Work out the finished part from the listing and answer in its coordinate system (mm). A direction names the side the tool comes from. Give positions to 0.01 mm unless a question says otherwise; leave off trailing zeros. Write each loop counter-clockwise with the first axis right and the second up, starting at its lowest first coordinate (ties: lowest second). Pieces come first, ordered by that corner, then holes.
1) Determine the mould class of faces 1 (the face through (-119.425, 112.175, 151.445)), 2 (the face through (-290.34, 195.39, 144.21)), 3 (the face through (6.177, -11.876, 49.783)), 4 (the face through (-272.86, 177.91, 127.75)) for opening direction Z: pulls with the +Z half, pulls with the -Z half, needs draft (parallel to the pull), parting line crosses it, or undercut.
2) Find section A-A (z = 58). Determine the outline of the cut face in (x, y).
3) Straight lines are drawn through the part: probe 1 along Y at (x, z) = (0, 34); probe 2 along X at (y, z) = (184.5, 133.5). For each, find the intervals that lie inside material, in ascending order.
4) A tool of negligible diameter and unlimited length cuts with its end or side. For faces 5 (the face through (-1, -14, 0)), 6 (the face through (16, 5, 50)), from which of +Z, -Z, +X, -X, +Y, -Y can it reach the whole face along a straight path? Write none if from no direction.
5) Given pin 1 Ø1 at (x, z) = (-27.5, 132) entering from -Y; pin 2 Ø6 at (x, y) = (-197, 204.5) entering from -Z (3 decimals), each flat-ended and moving along its own axis, determine where each tip first touches the part or whether it passes through.
```python
from build123d import *

# Parameters (mm, degrees)
PIPESKETCH_R    = 16.764
PIPESKETCH_R_2  = 13.3858
EXTRUSION_DEPTH = 95
SKETCH_3_R      = 16.764
SKETCH_3_R_2    = 13.3858
EXTRUDE_2_DEPTH = 5.980008255
SKETCH_4_R      = 16.764
SKETCH_4_R_2    = 13.3858
REVOLVE_2_ANGLE = 90
SKETCH_5_R      = 16.764
SKETCH_5_R_2    = 13.3858
EXTRUDE_3_DEPTH = 254.900237781
SKETCH_6_R      = 16.764
SKETCH_6_R_2    = 13.3858
REVOLVE_3_ANGLE = 90
SKETCH_7_R      = 16.764
SKETCH_7_R_2    = 13.3858
EXTRUDE_4_DEPTH = 58.9


with BuildPart() as part:
    # PipeSketch → Extrusion (new body)
    with BuildSketch(Plane.XY):
        Circle(PIPESKETCH_R)
        Circle(PIPESKETCH_R_2, mode=Mode.SUBTRACT)
    extrude(amount=EXTRUSION_DEPTH)

    # 草图3 → 凸台-拉伸2 (add)
    with BuildSketch(Plane.XY.offset(95)):
        Circle(SKETCH_3_R)
        Circle(SKETCH_3_R_2, mode=Mode.SUBTRACT)
    extrude(amount=EXTRUDE_2_DEPTH)

    # 草图4 → 旋转2 (revolve)
    with BuildSketch(Plane.XY.offset(100.980008255)):
        with Locations(Location((0, 0, 0), (0, 0, 315))):
            Circle(SKETCH_4_R)
        with Locations(Location((0, 0, 0), (0, 0, 315))):
            Circle(SKETCH_4_R_2, mode=Mode.SUBTRACT)
    revolve(axis=Axis((-26.940768363, 26.940768363, 100.980008255), (-0.7071067811865476, -0.7071067811865476, 0)), revolution_arc=REVOLVE_2_ANGLE)

    # 草图5 → 凸台-拉伸3 (add)
    with BuildSketch(Plane(origin=(-26.940768363, 26.940768363, 0), x_dir=(0.7071067811865475, 0.7071067811865477, 0), z_dir=(-0.7071067811865477, 0.7071067811865475, 0))):
        with Locations(Location((0, -139.080008255, 0), (0, 0, 270))):
            Circle(SKETCH_5_R)
        with Locations(Location((0, -139.080008255, 0), (0, 0, 270))):
            Circle(SKETCH_5_R_2, mode=Mode.SUBTRACT)
    extrude(amount=EXTRUDE_3_DEPTH)

    # 草图6 → 旋转3 (revolve)
    with BuildSketch(Plane(origin=(-207.182455024, 207.182455024, 0), x_dir=(0, 0, 1), z_dir=(-0.7071067811865476, 0.7071067811865476, 0))):
        with Locations(Location((139.080008255, 0, 0), (0, 0, 90))):
            Circle(SKETCH_6_R)
        with Locations(Location((139.080008255, 0, 0), (0, 0, 90))):
            Circle(SKETCH_6_R_2, mode=Mode.SUBTRACT)
    revolve(axis=Axis((-234.123223388, 180.241686661, 139.080008255), (0, 0, 1)), revolution_arc=REVOLVE_3_ANGLE)

    # 草图7 → 凸台-拉伸4 (add)
    with BuildSketch(Plane(origin=(-26.940768363, -26.940768363, 0), x_dir=(-0.7071067811865479, 0.7071067811865472, 0), z_dir=(-0.7071067811865472, -0.7071067811865479, 0))):
        with Locations((331.100237781, -139.080008255)):
            Circle(SKETCH_7_R)
        with Locations((331.100237781, -139.080008255)):
            Circle(SKETCH_7_R_2, mode=Mode.SUBTRACT)
    extrude(amount=EXTRUDE_4_DEPTH)


solid = part.part
```
Results:
1. face 1: undercut
1. face 2: undercut
1. face 3: needs draft
1. face 4: parting line crosses it
2. outline: circle Ø33.53 at (0, 0); hole circle Ø26.77 at (0, 0)
3. probe 1: y = -16.76 to -13.39, 13.39 to 16.76
3. probe 2: x = -306.1 to -300.95, -266.54 to -261.39, -206.86 to -201.71, -167.29 to -162.14
4. face 5: -Z, +X, -X, +Y, -Y
4. face 6: -Z
5. pin 1: stops at y = 3.66
5. pin 2: stops at z = 122.475
